Read the model definition and answer for the solid it produces. Units are mm, in the model's axes. Round coordinates to 2 decimals unless told otherwise and drop trailing zeros. Write each loop counter-clockwise with the first axis right and the second up, starting at its lowest first coordinate (ties: lowest second). Pieces come first, ordered by that corner, then holes. Notation, with made-up numbers: (5.5, 26.25) - (17.5, 26.25) arc R23 cw to (17.5, 58.25) - close; hole circle Ø1 at (-26, 1). An arc over 180 degrees is marked (long way). Answer as CSV lines item,"result". Start each with the question number.
1) Find section C-C on y = 310.5. Determine the outline of the cut face in (x, z), then the cut area to 3 significant figures.
2) Consider line 1 along Z through (x, y) = (6, 318); line 2 along Y through (x, z) = (11.25, -64.5); line 3 along Z through (x, y) = (15.5, 183.5). Determine where each line is inside the solid, lowest interval first.
3) Find section B-B on z = 170. Determine the outline of the cut face in (x, y).
4) Find section A-A on x = 5.5. Determine the outline of the cut face in (y, z), then the cut area to 3 significant figures.
5) Each of these flat-tipped pins is pushed along its axis until it touches: pin 1 (5.5 mm diameter, centred on x = 6, z = 15, fed in from +Y); pin 2 (8 mm diameter, centred on x = 14, y = -66, fed in from -Z); pin 3 (5.5 mm diameter, centred on x = 5, z = 492, fed in from -Y). Where does it stop, or does it pass through?
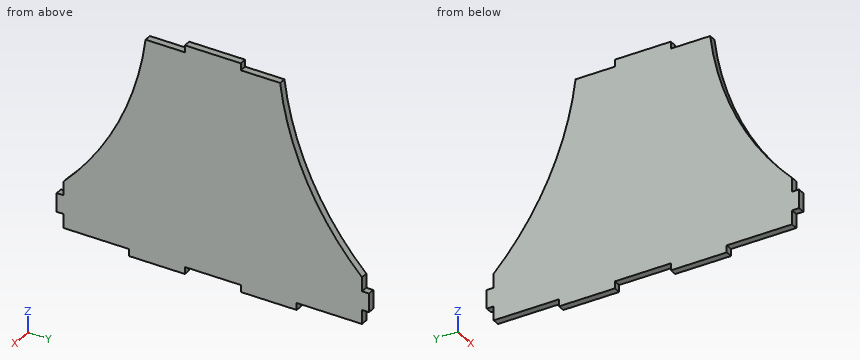
from build123d import *

# Parameters (mm, degrees)
F1_DEPTH = 19.05
F2_W     = 152.4
F2_H     = 19.05
F3_DEPTH = 19.05
F4_DEPTH = 19.05
F6_DEPTH = 19.051


with BuildPart() as f1:
    # F0 (on Right) → F1 (new body)
    with BuildSketch(Plane.YZ):
        with BuildLine():
            Line((-208.022948, 25.627738), (-208.022948, -101.372262))
            Line((-208.022948, -101.372262), (604.777052, -101.372262))
            Line((604.777052, -101.372262), (604.777052, 25.627738))
            ThreePointArc((604.777052, 25.627738), (429.785179, 293.978744), (376.177052, 609.827738))
            Line((376.177052, 609.827738), (198.377052, 609.827738))
            Line((198.377052, 609.827738), (20.577052, 609.827738))
            ThreePointArc((20.577052, 609.827738), (-33.031076, 293.978744), (-208.022948, 25.627738))
        make_face()
    extrude(amount=F1_DEPTH)

    # F2 (on face) → F3 (join)
    with BuildSketch(Plane.YZ.offset(19.05)):
        Polygon((274.577052, 628.877738), (198.377052, 628.877738), (122.177052, 628.877738), (122.177052, 609.827738), (274.577052, 609.827738), align=None)
        Polygon((-227.072948, -12.472262), (-227.072948, -37.872262), (-227.072948, -63.272262), (-208.022948, -63.272262), (-208.022948, -12.472262), align=None)
        with Locations((45.977052, -110.897262)):
            Rectangle(F2_W, F2_H)
        with Locations((350.777052, -110.897262)):
            Rectangle(F2_W, F2_H)
        Polygon((623.827052, -63.272262), (623.827052, -37.872262), (623.827052, -12.472262), (604.777052, -12.472262), (604.777052, -63.272262), align=None)
    extrude(amount=-F3_DEPTH)

    # F0 (on Right) → F4 (join)
    with BuildSketch(Plane.YZ):
        with BuildLine():
            Line((-208.022948, 25.627738), (-208.022948, -101.372262))
            Line((-208.022948, -101.372262), (604.777052, -101.372262))
            Line((604.777052, -101.372262), (604.777052, 25.627738))
            ThreePointArc((604.777052, 25.627738), (429.785179, 293.978744), (376.177052, 609.827738))
            Line((376.177052, 609.827738), (198.377052, 609.827738))
            Line((198.377052, 609.827738), (20.577052, 609.827738))
            ThreePointArc((20.577052, 609.827738), (-33.031076, 293.978744), (-208.022948, 25.627738))
        make_face()
    extrude(amount=F4_DEPTH)

    # F5 (on face) → F6 (cut, through all)
    with BuildSketch(Plane.YZ.offset(19.05)):
        with BuildLine():
            ThreePointArc((20.577052, 609.827738), (20.34373, 546.21452), (14.976085, 482.827738))
            Line((14.976085, 482.827738), (122.177052, 482.827738))
            Line((122.177052, 482.827738), (122.177052, 501.877738))
            Line((122.177052, 501.877738), (274.577052, 501.877738))
            Line((274.577052, 501.877738), (274.577052, 482.827738))
            Line((274.577052, 482.827738), (381.778018, 482.827738))
            ThreePointArc((381.778018, 482.827738), (376.410373, 546.21452), (376.177052, 609.827738))
            Line((376.177052, 609.827738), (274.577052, 609.827738))
            Line((274.577052, 609.827738), (274.577052, 628.877738))
            Line((274.577052, 628.877738), (122.177052, 628.877738))
            Line((122.177052, 628.877738), (122.177052, 609.827738))
            Line((122.177052, 609.827738), (20.577052, 609.827738))
        make_face()
    extrude(amount=-F6_DEPTH, mode=Mode.SUBTRACT)


solid = f1.part
Check values:
1,outline,"(0, -120.42) - (19.05, -120.42) - (19.05, 482.83) - (0, 482.83) - close"
1,area,"11,500 mm^2"
2,line 1,"z = -120.42 to 482.83"
2,line 2,"y = -208.02 to 604.78"
2,line 3,"z = -101.37 to 501.88"
3,outline,"(0, -94.61) - (19.05, -94.61) - (19.05, 491.37) - (0, 491.37) - close"
4,outline,"(-227.07, -63.27) - (-208.02, -63.27) - (-208.02, -101.37) - (-30.22, -101.37) - (-30.22, -120.42) - (122.18, -120.42) - (122.18, -101.37) - (274.58, -101.37) - (274.58, -120.42) - (426.98, -120.42) - (426.98, -101.37) - (604.78, -101.37) - (604.78, -63.27) - (623.83, -63.27) - (623.83, -12.47) - (604.78, -12.47) - (604.78, 25.63) arc R787.4 cw to (381.78, 482.83) - (274.58, 482.83) - (274.58, 501.88) - (122.18, 501.88) - (122.18, 482.83) - (14.98, 482.83) arc R787.4 cw to (-208.02, 25.63) - (-208.02, -12.47) - (-227.07, -12.47) - close"
4,area,"355,000 mm^2"
5,pin 1,"stops at y = 604.78"
5,pin 2,"stops at z = -101.37"
5,pin 3,"stops at y = 122.18"
